Check sheet for the modelled part. Datum: model origin and axes. Units: mm. Coordinates: 2 decimals unless noted, no trailing zeros. Write each loop counter-clockwise with the first axis right and the second up, starting at its lowest first coordinate (ties: lowest second). Pieces come first, ordered by that corner, then holes. Notation, with made-up numbers: (80.25, -4.5) - (136.25, -4.5) arc R12 cw to (136.25, 3.5) - close; hole circle Ø7 at (-2, 10.25). An arc over 180 degrees is marked (long way). Write each question's results on one line, items separated by ' | '.
from build123d import *

# Parameters (mm, degrees)
F0_R     = 11
F1_DEPTH = 3


with BuildPart() as f1:
    # F0 (on Top) → F1 (new body)
    with BuildSketch(Plane.XY):
        with BuildLine():
            Line((32.983547, 14.180062), (-32.983547, 14.180062))
            ThreePointArc((-32.983547, 14.180062), (-40.054615, 11.25113), (-42.983547, 4.180062))
            Line((-42.983547, 4.180062), (-42.983547, -4.180062))
            ThreePointArc((-42.983547, -4.180062), (-40.054615, -11.25113), (-32.983547, -14.180062))
            Line((-32.983547, -14.180062), (32.983547, -14.180062))
            ThreePointArc((32.983547, -14.180062), (40.054615, -11.25113), (42.983547, -4.180062))
            Line((42.983547, -4.180062), (42.983547, 4.180062))
            ThreePointArc((42.983547, 4.180062), (40.054615, 11.25113), (32.983547, 14.180062))
        make_face()
        with Locations((-26, 0)):
            Circle(F0_R, mode=Mode.SUBTRACT)
        Circle(F0_R, mode=Mode.SUBTRACT)
        with Locations((26, 0)):
            Circle(F0_R, mode=Mode.SUBTRACT)
    extrude(amount=F1_DEPTH)


solid = f1.part
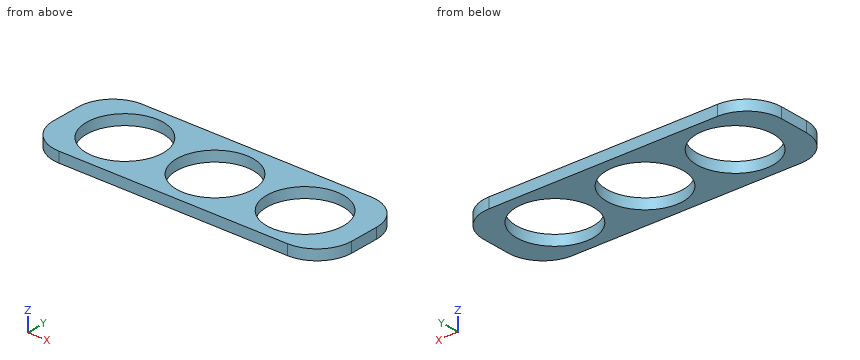
1. Sectioned sample at A-A (z = 1.75). Record the cut outline in (x, y), then the cut area to 3 significant figures.
Values follow:
outline: (-42.98, -4.18) arc R10 ccw to (-32.98, -14.18) - (32.98, -14.18) arc R10 ccw to (42.98, -4.18) - (42.98, 4.18) arc R10 ccw to (32.98, 14.18) - (-32.98, 14.18) arc R10 ccw to (-42.98, 4.18) - close; hole circle Ø22 at (-26, 0); hole circle Ø22 at (0, 0); hole circle Ø22 at (26, 0) | area: 1,210 mm^2
2. Sectioned sample at D-D (y = 8.5). Record the cut outline in (x, z), then the cut area to 3 significant figures.
Values follow:
outline: (-42, 0) - (-32.98, 0) - (-32.98, 3) - (-42, 3) - close; (-19.02, 0) - (-6.98, 0) - (-6.98, 3) - (-19.02, 3) - close; (6.98, 0) - (19.02, 0) - (19.02, 3) - (6.98, 3) - close; (32.98, 0) - (42, 0) - (42, 3) - (32.98, 3) - close | area: 126 mm^2
3. Material ranges on L1, parallel to Y at x = -26, z = 1.85; L2, parallel to X at y = -0.25, z = 1.05; L3, parallel to X at y = 2.25, z = 0.4, recorded low to high. Write a range as [from, to].
Values follow:
L1: y = [-14.18, -11], [11, 14.18] | L2: x = [-42.98, -37], [-15, -11], [11, 15], [37, 42.98] | L3: x = [-42.98, -36.77], [-15.23, -10.77], [10.77, 15.23], [36.77, 42.98]
4. Sectioned sample at B-B (y = 0). Record the cut outline in (x, z), then the cut area to 3 significant figures.
Values follow:
outline: (-42.98, 0) - (-37, 0) - (-37, 3) - (-42.98, 3) - close; (-15, 0) - (-11, 0) - (-11, 3) - (-15, 3) - close; (11, 0) - (15, 0) - (15, 3) - (11, 3) - close; (37, 0) - (42.98, 0) - (42.98, 3) - (37, 3) - close | area: 59.9 mm^2
5. Sectioned sample at C-C (x = 0). Record the cut outline in (y, z), then the cut area to 3 significant figures.
Values follow:
outline: (-14.18, 0) - (-11, 0) - (-11, 3) - (-14.18, 3) - close; (11, 0) - (14.18, 0) - (14.18, 3) - (11, 3) - close | area: 19.1 mm^2
